from build123d import *

# Parameters (mm, degrees)
F0_R      = 15.24
F1_DEPTH  = 12.7
F2_R      = 13.97
F3_DEPTH  = 12.192
F5_W      = 8.4936562926
F5_H      = 6.4059169963
F6_DEPTH  = 17.6276
F7_R      = 2.4085601445
F8_DEPTH  = 23.3426
F9_DEPTH  = 18.796
F10_R     = 2.0058104165
F11_DEPTH = 43.6118
F12_R     = 2.4085601445
F12_R_2   = 2.0058104165
F13_DEPTH = 25.4
F14_DEPTH = 16.1544
F15_DEPTH = 12.7762
F16_W     = 5.3624128923
F16_H     = 11.2610673532
F17_DEPTH = 25.4


with BuildPart() as f1:
    # F0 (on Front) → F1 (new body)
    with BuildSketch(Plane.XZ):
        Circle(F0_R)
    extrude(amount=F1_DEPTH)

    # F2 (on face) → F3 (cut)
    with BuildSketch(Plane(origin=(0, 0, 0), x_dir=(-1, 0, 0), z_dir=(0, 1, 0))):
        Circle(F2_R)
    extrude(amount=-F3_DEPTH, mode=Mode.SUBTRACT)

    # F5 (on offset) → F6 (cut)
    with BuildSketch(Plane.YZ.offset(31.75)):
        with Locations((-6.6680489108, 0)):
            Rectangle(F5_W, F5_H)
    extrude(amount=-F6_DEPTH, mode=Mode.SUBTRACT)

    # F7 (on offset) → F8 (join)
    with BuildSketch(Plane.YZ.offset(31.75)):
        with Locations((-6.3897143118, 0)):
            Circle(F7_R)
    extrude(amount=-F8_DEPTH)

    # F9 (add): a face of the model
    f9_faces = [f1.faces().sort_by_distance(p)[0] for p in [
        (31.75, -6.3897143118, 0),
    ]]
    extrude(f9_faces, amount=F9_DEPTH)

    # F10 (on face) → F11 (cut)
    with BuildSketch(Plane.YZ.offset(50.546)):
        with Locations((-6.3897143118, 0)):
            Circle(F10_R)
    extrude(amount=-F11_DEPTH, mode=Mode.SUBTRACT)

    # F12 (on face) → F13 (join)
    with BuildSketch(Plane.YZ.offset(50.546)):
        with Locations((-6.3897143118, 0)):
            Circle(F12_R)
        with Locations((-6.3897143118, 0)):
            Circle(F12_R_2, mode=Mode.SUBTRACT)
    extrude(amount=F13_DEPTH)

    # F14 (cut): a face of the model
    f14_faces = [f1.faces().sort_by_distance(p)[0] for p in [
        (75.946, -8.7301500879, 0),
    ]]
    extrude(f14_faces, amount=-F14_DEPTH, mode=Mode.SUBTRACT)

    # F15 (add): a face of the model
    f15_faces = [f1.faces().sort_by_distance(p)[0] for p in [
        (59.7916, -8.7301500879, 0),
    ]]
    extrude(f15_faces, amount=F15_DEPTH)

    # F16 (on face) → F17 (cut)
    with BuildSketch(Plane.XZ.offset(12.7)):
        with Locations((-9.5757367089, 0)):
            Rectangle(F16_W, F16_H)
    extrude(amount=-F17_DEPTH, mode=Mode.SUBTRACT)


solid = f1.part
The listing builds one solid part. Answer for the finished solid, in the listing's coordinates (mm). A direction names the side the tool comes from. Round coordinates to 2 decimals unless told otherwise and drop trailing zeros. Write each loop counter-clockwise with the first axis right and the second up, starting at its lowest first coordinate (ties: lowest second). Pieces come first, ordered by that corner, then holes. Notation, with made-up numbers: (-38, 19.25) - (-22, 19.25) arc R17 ccw to (-22, 32.25) - close; hole circle Ø8 at (-15.5, 80.5). An arc over 180 degrees is marked (long way). Use one line per item in the form item = value. Start each with the question number.
Item 1: A tool of negligible diameter and unlimited length cuts with its end or side. For faces 4 (the flat face through (0, -12.7, 0)), 5 (the cylindrical face through (42.94, -4.09, 0.72)), 6 (the cylindrical face through (11.23, -4.09, 0.72)), from which of +Z, -Z, +X, -X, +Y, -Y can it reach the whole face along a straight path? Write none if from no direction.
Item 2: A cutting plane is placed at B-B (x = 0). Write down the section's boundary in (y, z).
Item 3: Flat-ended cylindrical pins translate along their axes: pin 1 Ø5 at (x, y) = (8, -1.5) entering from +Z; pin 2 Ø12 at (x, z) = (32, -1) entering from -Y; pin 3 Ø5 at (y, z) = (-8.5, 9.5) entering from -X. Find the tip coordinate at first contact, or state that the pin passes through.
Item 4: A cutting plane is placed at A-A (z = 0). Write down the section's boundary in (x, y), plus the area to 3 significant figures.
Item 5: A cutting plane is placed at C-C (x = 35). Write down the section's boundary in (y, z).
Item 6: Determine the mould class of faces 1 (the flat face through (13.5, 0, -4.4)), 2 (the cylindrical face through (-13.325, -6.011, 4.196)), 3 (the cylindrical face through (-3.3, -6.26, -14.88)) for opening direction X: +X half, -X half, draft (parallel to the pull), parting line (faces both ways), or undercut.
Item 7: A cutting plane is placed at D-D (y = -6.25). Write down the section's boundary in (x, z).
Item 8: Find the intervals of material crossed by line 1 (Z direction, x = 0, y = -9.5); line 2 (Z direction, x = 46, y = -6.25); line 3 (X direction, y = -6.75, z = 6.5), in increasing order. Write a range as [from, to].
The answers:
q1.face_4 = +Z, -Z, +X, -X, -Y
q1.face_5 = +X
q1.face_6 = none
q2.outline = (-12.7, -15.24) - (0, -15.24) - (0, -13.97) - (-12.19, -13.97) - (-12.19, 13.97) - (0, 13.97) - (0, 15.24) - (-12.7, 15.24) - close
q3.pin_1 = 14.21
q3.pin_2 = -8.8
q3.pin_3 = -13.54
q4.outline = (-15.24, -12.7) - (-12.26, -12.7) - (-12.26, -12.19) - (-13.97, -12.19) - (-13.97, 0) - (-15.24, 0) - close; (-6.89, -12.7) - (15.24, -12.7) - (15.24, -10.91) - (14.12, -10.91) - (14.12, -8.8) - (72.57, -8.8) - (72.57, -8.4) - (8.41, -8.4) - (8.41, -8.8) - (13.97, -8.8) - (13.97, -12.19) - (-6.89, -12.19) - close; (8.41, -4.38) - (72.57, -4.38) - (72.57, -3.98) - (14.12, -3.98) - (14.12, -2.42) - (15.24, -2.42) - (15.24, 0) - (13.97, 0) - (13.97, -3.98) - (8.41, -3.98) - close
q4.area = 85.2 mm^2
q5.outline = circle Ø4.82 at (-6.39, 0); hole circle Ø4.01 at (-6.39, 0)
q6.face_1 = draft
q6.face_2 = undercut
q6.face_3 = parting line
q7.outline = (8.41, -2.4) - (13.76, -2.4) arc R13.97 cw (long way) to (13.76, 2.4) - (8.41, 2.4) - (8.41, 2) - (72.57, 2) - (72.57, 2.4) - (14.12, 2.4) - (14.12, 3.2) - (14.9, 3.2) arc R15.24 ccw (long way) to (14.9, -3.2) - (14.12, -3.2) - (14.12, -2.4) - (72.57, -2.4) - (72.57, -2) - (8.41, -2) - close
q8.line_1 = [-15.24, -13.97], [13.97, 15.24]
q8.line_2 = [-2.4, -2], [2, 2.4]
q8.line_3 = [-13.78, -12.37], [12.37, 13.78]
